```python
from build123d import *

# Parameters (mm, degrees)
F1_DEPTH = 5
F2_R     = 8
F3_DEPTH = 5
F6_R     = 1
F7_DEPTH = 3
F8_R     = 1


with BuildPart() as f1:
    # F0 (on Front) → F1 (new body)
    with BuildSketch(Plane.XZ):
        Polygon((24.537386, -42.5), (49.074773, 0), (24.537386, 42.5), (-24.537386, 42.5), (-49.074773, 0), (-24.537386, -42.5), align=None)
    extrude(amount=F1_DEPTH)

    # F2 (on face) → F3 (cut)
    with BuildSketch(Plane.XZ.offset(5)):
        Circle(F2_R)
    extrude(amount=-F3_DEPTH, mode=Mode.SUBTRACT)

    # F6 (on face) → F7 (join)
    with BuildSketch(Plane.XZ.offset(5)):
        with Locations((-22.990381, 39.820508)):
            Circle(F6_R)
        with Locations((22.990381, -39.820508)):
            Circle(F6_R)
    extrude(amount=F7_DEPTH)

    # F8
    f8_edges = [f1.edges().sort_by_distance(p)[0] for p in [
        (-23.990381, -8, 39.820508),
        (21.990381, -8, -39.820508),
    ]]
    fillet(f8_edges, radius=F8_R)


solid = f1.part
```
Build history of the part. All positions in model axes, mm. A direction names the side the tool comes from. Give positions to 0.01 mm unless a question says otherwise; leave off trailing zeros. Loops run counter-clockwise (first coordinate to the right, second up) from the corner with the lowest first, then second, coordinate; pieces in that order, holes last. Notation, with made-up numbers: (-20, 17.5) - (11, 17.5) arc R12 ccw to (11, 28.5) - close; hole circle Ø6 at (-30.75, -11.75). An arc over 180 degrees is marked (long way). Use a Markdown table: item, result.
(1) Pull direction X, two halves, no side cores. Call faces 1 (the face through (0, -2, 42.5)), 2 (the face through (-1.73, -2.54, -7.81)), 3 (the face through (36.98, -2.46, 20.95)): +X half, -X half, draft (parallel to the pull), parting line (faces both ways), or undercut.
Taken from the geometry:
| item | result |
|---|---|
| face 1 | draft |
| face 2 | undercut |
| face 3 | +X half |
(2) Which spindle directions (+Z, -Z, +X, -X, +Y, -Y) get a long thin tool onto all of the face, cutting with end or side? Do faces 4 (the face through (-23.207, -5.986, 38.844)), 5 (the face through (0, -2, -42.5)). Say none if no direction does.
Taken from the geometry:
| item | result |
|---|---|
| face 4 | -Y |
| face 5 | -Z, +X, -X, +Y, -Y |
(3) Band-saw the part on C-C (x = -20.5). Give the cut face in (y, z), and give its area (3 significant figures).
Taken from the geometry:
| item | result |
|---|---|
| outline | (-5, -42.5) - (0, -42.5) - (0, 42.5) - (-5, 42.5) - close |
| area | 425 mm2 |
(4) Band-saw the part on B-B (y = -3.5). Give the cut face in (x, z).
Taken from the geometry:
| item | result |
|---|---|
| outline | (-49.07, 0) - (-24.54, -42.5) - (24.54, -42.5) - (49.07, 0) - (24.54, 42.5) - (-24.54, 42.5) - close; hole circle Ø16 at (0, 0) |
(5) Drop flat-ended pins along their axis: pin 1 Ø3 at (y, z) = (-2, 6) entering from -X; pin 2 Ø1 at (y, z) = (-4.5, 20.5) entering from +X; pin 3 Ø2 at (y, z) = (-3.5, 22) entering from +X. Give the stop position or say it passes through.
Taken from the geometry:
| item | result |
|---|---|
| pin 1 | x = -46.48 |
| pin 2 | x = 37.53 |
| pin 3 | x = 36.95 |
(6) Band-saw the part on D-D (z = -13.5). Give the cut face in (x, y), and give its area (3 significant figures).
Taken from the geometry:
| item | result |
|---|---|
| outline | (-41.28, -5) - (41.28, -5) - (41.28, 0) - (-41.28, 0) - close |
| area | 413 mm2 |
(7) Band-saw the part on A-A (x = 0). Give the cut face in (y, z).
Taken from the geometry:
| item | result |
|---|---|
| outline | (-5, -42.5) - (0, -42.5) - (0, -8) - (-5, -8) - close; (-5, 8) - (0, 8) - (0, 42.5) - (-5, 42.5) - close |
(8) Wall check: line 1 along Z through (x, y) = (0, -1.75); line 2 along Y through (x, z) = (-3, -35.5); line 3 along X through (y, z) = (-3.25, 4). Give the ranges that are in metal, low to high.
Taken from the geometry:
| item | result |
|---|---|
| line 1 | -42.5 to -8, 8 to 42.5 |
| line 2 | -5 to 0 |
| line 3 | -46.77 to -6.93, 6.93 to 46.77 |
